Design review of the part built by this model. Coordinates are the model's own, in mm. Face numbers are marked on the shaded views. A direction names the side the tool comes from. Give positions to 0.01 mm unless a question says otherwise; leave off trailing zeros. Write each loop counter-clockwise with the first axis right and the second up, starting at its lowest first coordinate (ties: lowest second). Pieces come first, ordered by that corner, then holes. Notation, with made-up numbers: (49.5, 19) -> (93.5, 19) arc R5 ccw to (93.5, 23) -> close; hole circle Ø9 at (89, 74.5). An arc over 180 degrees is marked (long way). Write each question's results on one line, items separated by ' | '. Start each with the question number.
(1) Take a section at C-C (x = 33.5). State the section outline as (y, z) points.
(2) Take a section at B-B (y = 0). Count the separate pieces of the cut face and the enclosed holes in it, plus the area to 3 significant figures.
(3) Clearance check with flat-ended pins moving along their axes: pin 1 (6 mm diameter, centred on x = 70.5, z = 19.5, fed in from -Y); pin 2 (0.6 mm diameter, centred on x = 74, y = -1, fed in from +Z); pin 3 (1.2 mm diameter, centred on y = 1.5, z = 2, fed in from +X). State where each tip first meets the part, or that it passes through.
(4) To check wall thickness, follow probe 1 along Y at (x, z) = (33.5, 16.5); probe 2 along Z at (x, y) = (20, -4); probe 3 along Z at (x, y) = (18, 2). State the ranges of each line that lie inside material, in increasing order.
(5) Mouldability with a two-part tool opening along Z and no side actions: class the marked faces 1, 2 and 3 as released by +Z, released by -Z, zero draft, split by the parting line, or undercut.
(6) Take a section at A-A (x = 70.5). State the section outline as (y, z) points, plus the area to 3 significant figures.
(7) For the marked faces 4, 5 and 6, list the 3-axis set-ups (+Z, -Z, +X, -X, +Y, -Y) from which the entire face can be reached by the end or side of a thin tool; tool diameter is ignored.
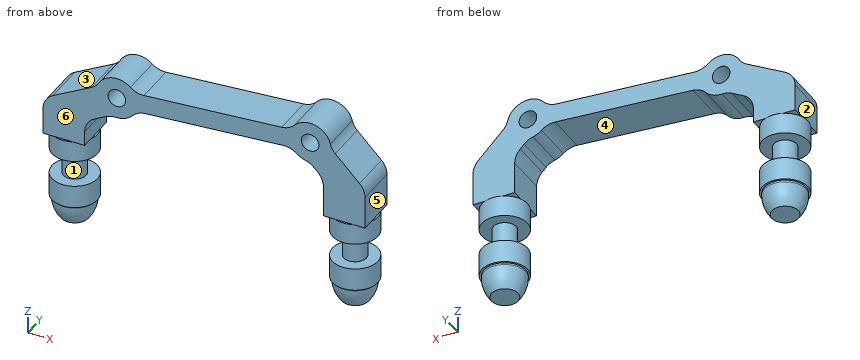
from build123d import *

# Parameters (mm, degrees)
SKETCH1_R           = 2.328285793
BOSS_EXTRUDE1_DEPTH = 5.5
FILLET1_R           = 5
SKETCH3_R           = 6
BOSS_EXTRUDE2_DEPTH = 5.5
SKETCH4_R           = 3
BOSS_EXTRUDE3_DEPTH = 7
LPATTERN1_COUNT     = 2
LPATTERN1_PITCH     = 74


with BuildPart() as part:
    # Sketch1 → Boss-Extrude1 (new, symmetric)
    with BuildSketch(Plane(origin=(0, 0, 0), x_dir=(1, 0, 0), z_dir=(0, 1, 0))):
        with BuildLine():
            Line((0, 0), (11, 0))
            Line((11, 0), (11, -6.854633107))
            Line((11, -6.854633107), (18.08275142, -10.685735567))
            ThreePointArc((18.08275142, -10.685735567), (21.90921539, -11.055742603), (24.558649677, -13.841281989))
            Line((24.558649677, -13.841281989), (65.78368238, -16.6704509))
            ThreePointArc((65.78368238, -16.6704509), (67.721094199, -14.75366641), (70.340842438, -14.002303312))
            Line((70.340842438, -14.002303312), (74, -10.343145751))
            Line((74, -10.343145751), (74, 0))
            Line((74, 0), (85, 0))
            Line((85, 0), (85, -10.656854249))
            Line((85, -10.656854249), (75.997696688, -19.659157562))
            ThreePointArc((75.997696688, -19.659157562), (71.523597121, -24.903910522), (65.441350323, -21.658718011))
            Line((65.441350323, -21.658718011), (24.21631762, -18.8295491))
            ThreePointArc((24.21631762, -18.8295491), (18.891090881, -21.466189686), (14.276625407, -17.722311778))
            Line((14.276625407, -17.722311778), (0, -10))
            Line((0, -10), (0, 0))
        make_face()
        with Locations(Location((19.5, -16, 0), (0, 0, 270))):
            Circle(SKETCH1_R, mode=Mode.SUBTRACT)
        with Locations(Location((70.5, -19.5, 0), (0, 0, 270))):
            Circle(SKETCH1_R, mode=Mode.SUBTRACT)
    extrude(amount=BOSS_EXTRUDE1_DEPTH, both=True)

    # Fillet1
    fillet1_edges = [part.edges().sort_by_distance(p)[0] for p in [
        (11, 0, 6.854633107),
        (18.08275142, 0, 10.685735567),
        (24.558649677, 0, 13.841281989),
        (65.78368238, 0, 16.6704509),
        (70.340842438, 0, 14.002303312),
        (74, 0, 10.343145751),
        (85, 0, 10.656854249),
        (75.997696688, 0, 19.659157562),
        (65.441350323, 0, 21.658718011),
        (24.21631762, 0, 18.8295491),
        (14.276625407, 0, 17.722311778),
        (0, 0, 10),
    ]]
    fillet(fillet1_edges, radius=FILLET1_R)

    # Sketch3 → Boss-Extrude2 (add)
    with BuildSketch(Plane(origin=(0, 0, 0), x_dir=(-1, 0, 0), z_dir=(0, 0, -1))):
        with Locations(Location((-79.5, 0, 0), (0, 0, 156.443535691))):
            Circle(SKETCH3_R)
        with Locations(Location((-5.5, 0, 0), (0, 0, 156.443535691))):
            Circle(SKETCH3_R)
    extrude(amount=BOSS_EXTRUDE2_DEPTH)

    # Sketch4 → Boss-Extrude3 (add)
    with BuildSketch(Plane(origin=(0, 0, -5.5), x_dir=(-1, 0, 0), z_dir=(0, 0, -1))):
        with Locations((-79.5, 0)):
            Circle(SKETCH4_R)
        with Locations((-5.5, 0)):
            Circle(SKETCH4_R)
    extrude(amount=BOSS_EXTRUDE3_DEPTH)

    # Sketch5 → Revolve1 (revolve)
    with BuildSketch(Plane(origin=(0, 0, 0), x_dir=(1, 0, 0), z_dir=(0, 1, 0)), mode=Mode.PRIVATE) as revolve1_sk:
        with BuildLine():
            Line((5.5, 12.5), (11.5, 12.5))
            Line((11.5, 12.5), (11.5, 18.5))
            Line((11.5, 18.5), (11, 18.5))
            Line((11, 18.5), (11, 19))
            ThreePointArc((11, 19), (10.484481189, 21.926174978), (9, 24.5))
            Line((9, 24.5), (5.5, 24.5))
            Line((5.5, 24.5), (5.5, 12.5))
        make_face()
    revolve1 = revolve(revolve1_sk.sketch.rotate(Axis((5.5, 0, -12.5), (0, 0, 1)), 180), axis=Axis((5.5, 0, -12.5), (0, 0, 1)))

    # LPattern1: Revolve1 ×2
    with Locations(*[(i * LPATTERN1_PITCH, 0, 0) for i in range(1, LPATTERN1_COUNT)]):
        add(revolve1)


solid = part.part
Report:
1) outline: (-5.5, 14.45) -> (5.5, 14.45) -> (5.5, 19.47) -> (-5.5, 19.47) -> close
2) separate pieces: 1 | enclosed holes: 2 | area: 1,200 mm2
3) pin 1: y = -5.5 | pin 2: z = 23.97 | pin 3: x = 85
4) probe 1: -5.5 to 5.5 | probe 2: 10.52 to 13.73, 18.27 to 21.48 | probe 3: 10.4 to 14.22, 17.78 to 21.29
5) face 1: undercut | face 2: zero draft | face 3: released by +Z
6) outline: (-5.5, 13.62) -> (5.5, 13.62) -> (5.5, 17.17) -> (-5.5, 17.17) -> close; (-5.5, 21.83) -> (5.5, 21.83) -> (5.5, 25) -> (-5.5, 25) -> close | area: 74.0 mm2
7) face 4: -Z, +Y, -Y | face 5: +Z, +X, +Y, -Y | face 6: +Z, +X, -X, -Y
